The listing builds one solid part. Answer for the finished solid, in the listing's coordinates (mm). Round coordinates to 2 decimals unless told otherwise and drop trailing zeros. Loops run counter-clockwise (first coordinate to the right, second up) from the corner with the lowest first, then second, coordinate; pieces in that order, holes last. Notation, with made-up numbers: (89.5, 63) - (103.5, 63) arc R15 ccw to (103.5, 91) - close; hole circle Ø3 at (74.5, -0.5). An arc over 180 degrees is marked (long way). Write item = value, one per line. Start each with the question number.
1) Straight lines are drawn through the part: line 1 along Y through (x, z) = (6.25, 0.1); line 2 along X through (y, z) = (7, 1.4); line 3 along Y through (x, z) = (-6.5, 1.45). For each, find the intervals that lie inside material, in ascending order.
2) Section B-B, the plane x = -8 is taken. Determine the outline of the cut face in (y, z), and give its area (3 significant figures).
3) Given pin 1 Ø1.2 at (x, y) = (13, 2.5) entering from -Z; pin 2 Ø6.5 at (x, y) = (5.97, -17.2) entering from -Z, each flat-ended and moving along its own axis, determine where each tip first touches the part or whether it passes through.
4) Section A-A, the plane y = 2.5 is taken. Determine the outline of the cut face in (x, z), and give its area (4 significant figures).
5) Section C-C, the plane y = 23.5 is taken. Determine the outline of the cut face in (x, z).
6) Section D-D, the plane z = 1.25 is taken. Determine the outline of the cut face in (x, y).
from build123d import *
from build123d import SkipClean  # not in build123d's __all__

# Parameters (mm, degrees)
F0_W     = 10.5
F0_H     = 5
F0_R     = 1
F0_R_2   = 2
F1_DEPTH = 1.5
F2_R     = 2
F4_DEPTH = 1.5
F3_R     = 1
F5_DEPTH = 1.5


with BuildPart() as f1:
    # F0 (on Top) → F1 (new body)
    with BuildSketch(Plane.XY):
        with Locations((-5.25, 23.5)):
            Rectangle(F0_W, F0_H)
        with Locations((-8, 23.5)):
            Circle(F0_R, mode=Mode.SUBTRACT)
        Polygon((8.75, 21), (0, 21), (8.75, 12.25), align=None)
        Polygon((8.75, 2.5), (8.75, 0), (15.5, 0), (15.5, 26), (0, 26), (0, 21), (8.75, 21), (8.75, 12.25), align=None)
        with Locations((13, 2.5)):
            Circle(F0_R, mode=Mode.SUBTRACT)
        with Locations((13, 23.5)):
            Circle(F0_R, mode=Mode.SUBTRACT)
        Polygon((15.5, 0), (8.75, 0), (2.5261364178, -17.8039236821), (3.1339050396, -21.2507508176), (10.0275593107, -20.035213574), align=None)
        with Locations((5.9729635533, -17.1961550602)):
            Circle(F0_R_2, mode=Mode.SUBTRACT)
    extrude(amount=F1_DEPTH)

    # F2
    f2_edges = [f1.edges().sort_by_distance(p)[0] for p in [
        (3.133905, -21.250751, 0.75),
        (2.526136, -17.803924, 0.75),
        (10.027559, -20.035214, 0.75),
        (0, 21, 0.75),
        (8.75, 12.25, 0.75),
        (8.75, 0, 0.75),
        (15.5, 0, 0.75),
        (-10.5, 21, 0.75),
        (-10.5, 26, 0.75),
        (15.5, 26, 0.75),
    ]]
    fillet(f2_edges, radius=F2_R)

    # F3 (on face) → F4 (cut, through all)
    with BuildSketch(Plane.XY.offset(1.5)):
        with BuildLine():
            Line((15.4293248166, -0.2587497013), (9.7925199679, -18.3840055542))
            ThreePointArc((9.7925199679, -18.3840055542), (9.2828500145, -19.4421852503), (8.4878041885, -20.3067139457))
            Line((8.4878041885, -20.3067139457), (8.7794635144, -20.2552865373))
            ThreePointArc((8.7794635144, -20.2552865373), (9.7797768114, -19.7634897702), (10.3614919757, -18.8126489739))
            Line((10.3614919757, -18.8126489739), (15.4293248166, -0.2587497013))
        make_face()
        with BuildLine():
            ThreePointArc((2.9760281468, -19.8453772421), (3.6090713176, -20.5721430448), (4.5085212955, -20.9184404971))
            ThreePointArc((4.5085212955, -20.9184404971), (3.6786578079, -20.4727632374), (2.9760281468, -19.8453772421))
        make_face()
    extrude(amount=-F4_DEPTH, mode=Mode.SUBTRACT)

    # F3 (on face) → F5 (join)
    with BuildSketch(Plane.XY.offset(1.5)):
        with BuildLine():
            ThreePointArc((2.2760890833, -15.6686999373), (2.9532568393, -14.5729182502), (3.9435858611, -13.7491815787))
            Line((3.9435858611, -13.7491815787), (8.6379648829, -0.3204865672))
            ThreePointArc((8.6379648829, -0.3204865672), (8.6665084457, -0.2323302993), (8.6909380974, -0.1429465499))
            Line((8.6909380974, -0.1429465499), (2.2760890833, -15.6686999373))
        make_face()
        with BuildLine():
            Line((2.6984727346, -17.3109400888), (3.9435858611, -13.7491815787))
            ThreePointArc((3.9435858611, -13.7491815787), (2.9532568393, -14.5729182502), (2.2760890833, -15.6686999373))
            ThreePointArc((2.2760890833, -15.6686999373), (2.027975468, -17.8572670075), (2.9760281468, -19.8453772421))
            ThreePointArc((2.9760281468, -19.8453772421), (2.8602115576, -19.570341978), (2.7866086843, -19.2811353116))
            Line((2.7866086843, -19.2811353116), (2.6168221115, -18.3182278083))
            ThreePointArc((2.6168221115, -18.3182278083), (2.5929761176, -17.8093417002), (2.6984727346, -17.3109400888))
        make_face()
        with BuildLine():
            ThreePointArc((4.5085212955, -20.9184404971), (6.5807353289, -21.1497121256), (8.4878041885, -20.3067139457))
            Line((8.4878041885, -20.3067139457), (5.1035205457, -20.9034544623))
            ThreePointArc((5.1035205457, -20.9034544623), (4.8065815101, -20.9332048908), (4.5085212955, -20.9184404971))
        make_face()
        with BuildLine():
            ThreePointArc((9.9729635533, -17.1961550602), (9.927595373, -17.7968939144), (9.7925199679, -18.3840055542))
            Line((9.7925199679, -18.3840055542), (15.4293248166, -0.2587497013))
            ThreePointArc((15.4293248166, -0.2587497013), (15.4822524604, 0.0023801957), (15.5, 0.2682282413))
            Line((15.5, 0.2682282413), (15.5, 24))
            ThreePointArc((15.5, 24), (14.9142135624, 25.4142135624), (13.5, 26))
            Line((13.5, 26), (-8.5, 26))
            ThreePointArc((-8.5, 26), (-9.9142135624, 25.4142135624), (-10.5, 24))
            Line((-10.5, 24), (-10.5, 23))
            ThreePointArc((-10.5, 23), (-9.9142135624, 21.5857864376), (-8.5, 21))
            Line((-8.5, 21), (-0.8284271247, 21))
            ThreePointArc((-0.8284271247, 21), (-0.06306026, 20.847759065), (0.5857864376, 20.4142135624))
            Line((0.5857864376, 20.4142135624), (8.1642135624, 12.8357864376))
            ThreePointArc((8.1642135624, 12.8357864376), (8.597759065, 12.18693974), (8.75, 11.4215728753))
            Line((8.75, 11.4215728753), (8.75, 0.339504797))
            ThreePointArc((8.75, 0.339504797), (8.7351796134, 0.0964782499), (8.6909380974, -0.1429465499))
            ThreePointArc((8.6909380974, -0.1429465499), (8.6665084457, -0.2323302993), (8.6379648829, -0.3204865672))
            Line((8.6379648829, -0.3204865672), (3.9435858611, -13.7491815787))
            ThreePointArc((3.9435858611, -13.7491815787), (7.9582203668, -13.7235831914), (9.9729635533, -17.1961550602))
        make_face()
        with Locations((-8, 23.5)):
            Circle(F3_R, mode=Mode.SUBTRACT)
        with Locations((13, 2.5)):
            Circle(F3_R, mode=Mode.SUBTRACT)
        with Locations((13, 23.5)):
            Circle(F3_R, mode=Mode.SUBTRACT)
    with SkipClean():  # cleaning this boolean's faces spoils the solid; the shape is the same uncleaned
        extrude(amount=-F5_DEPTH)


solid = f1.part
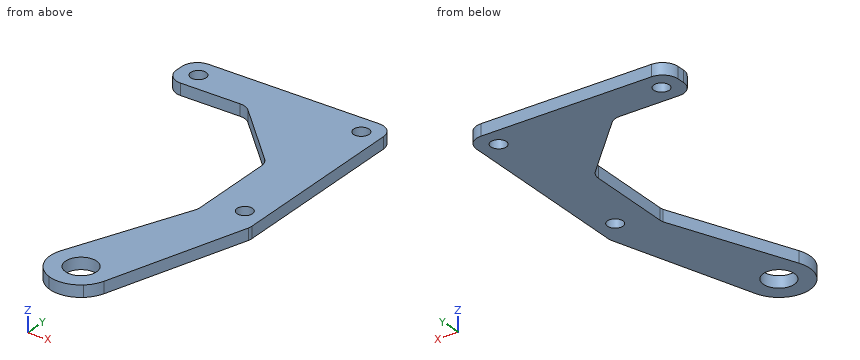
Geometry check:
q1.line_1 = -21.19 to -19.18, -15.22 to -6.05, 14.75 to 26
q1.line_2 = 8.75 to 15.5
q1.line_3 = 21 to 26
q2.outline = (21, 0) - (22.5, 0) - (22.5, 1.5) - (21, 1.5) - close; (24.5, 0) - (26, 0) - (26, 1.5) - (24.5, 1.5) - close
q2.area = 4.50 mm2
q3.pin_1 = through
q3.pin_2 = 0
q4.outline = (8.75, 0) - (12, 0) - (12, 1.5) - (8.75, 1.5) - close; (14, 0) - (15.5, 0) - (15.5, 1.5) - (14, 1.5) - close
q4.area = 7.125 mm2
q5.outline = (-10.5, 0) - (-9, 0) - (-9, 1.5) - (-10.5, 1.5) - close; (-7, 0) - (12, 0) - (12, 1.5) - (-7, 1.5) - close; (14, 0) - (15.5, 0) - (15.5, 1.5) - (14, 1.5) - close
q6.outline = (-10.5, 23) arc R2 ccw to (-8.5, 21) - (-0.83, 21) arc R2 cw to (0.59, 20.41) - (8.16, 12.84) arc R2 cw to (8.75, 11.42) - (8.75, 0.34) arc R2 cw to (8.69, -0.14) - (2.28, -15.67) arc R4 ccw (long way) to (9.79, -18.38) - (15.43, -0.26) arc R2 ccw to (15.5, 0.27) - (15.5, 24) arc R2 ccw to (13.5, 26) - (-8.5, 26) arc R2 ccw to (-10.5, 24) - close; hole circle Ø2 at (-8, 23.5); hole circle Ø4 at (5.97, -17.2); hole circle Ø2 at (13, 2.5); hole circle Ø2 at (13, 23.5)
